```python
from build123d import *

# Parameters (mm, degrees)
SKETCH1_R           = 16
BOSS_EXTRUDE1_DEPTH = 1.6
SKETCH2_W           = 5
SKETCH2_H           = 6.5
BOSS_EXTRUDE2_DEPTH = 1.2
CUT_EXTRUDE1_DEPTH  = 23.683915006
SKETCH4_W           = 11.5
SKETCH4_H           = 5
BOSS_EXTRUDE3_DEPTH = 4.4


with BuildPart() as part:
    # Sketch1 → Boss-Extrude1 (new body)
    with BuildSketch(Plane.XY):
        Circle(SKETCH1_R)
    extrude(amount=BOSS_EXTRUDE1_DEPTH)

    # Sketch2 → Boss-Extrude2 (add)
    with BuildSketch(Plane.XY.offset(1.6)):
        Rectangle(SKETCH2_W, SKETCH2_H)
    extrude(amount=BOSS_EXTRUDE2_DEPTH)

    # Sketch3 → Cut-Extrude1 (cut, through all)
    with BuildSketch(Plane.XY.offset(1.6)):
        with BuildLine():
            Line((-5.656854249, -7.778174593), (-8.838834765, -10.960155108))
            ThreePointArc((-8.838834765, -10.960155108), (-10.960155108, -10.960155108), (-10.960155108, -8.838834765))
            Line((-10.960155108, -8.838834765), (-7.778174593, -5.656854249))
            ThreePointArc((-7.778174593, -5.656854249), (-5.656854249, -5.656854249), (-5.656854249, -7.778174593))
        make_face()
        with BuildLine():
            Line((-9.5, -1.5), (-11.5, -1.5))
            ThreePointArc((-11.5, -1.5), (-13, 0), (-11.5, 1.5))
            Line((-11.5, 1.5), (-9.5, 1.5))
            ThreePointArc((-9.5, 1.5), (-8, 0), (-9.5, -1.5))
        make_face()
        with BuildLine():
            Line((-7.778174593, 5.656854249), (-10.960155108, 8.838834765))
            ThreePointArc((-10.960155108, 8.838834765), (-10.960155108, 10.960155108), (-8.838834765, 10.960155108))
            Line((-8.838834765, 10.960155108), (-5.656854249, 7.778174593))
            ThreePointArc((-5.656854249, 7.778174593), (-5.656854249, 5.656854249), (-7.778174593, 5.656854249))
        make_face()
        with BuildLine():
            Line((5.656854249, 7.778174593), (8.838834765, 10.960155108))
            ThreePointArc((8.838834765, 10.960155108), (10.960155108, 10.960155108), (10.960155108, 8.838834765))
            Line((10.960155108, 8.838834765), (7.778174593, 5.656854249))
            ThreePointArc((7.778174593, 5.656854249), (5.656854249, 5.656854249), (5.656854249, 7.778174593))
        make_face()
        with BuildLine():
            Line((7.778174593, -5.656854249), (10.960155108, -8.838834765))
            ThreePointArc((10.960155108, -8.838834765), (10.960155108, -10.960155108), (8.838834765, -10.960155108))
            Line((8.838834765, -10.960155108), (5.656854249, -7.778174593))
            ThreePointArc((5.656854249, -7.778174593), (5.656854249, -5.656854249), (7.778174593, -5.656854249))
        make_face()
        with BuildLine():
            Line((9.5, 1.5), (11.5, 1.5))
            ThreePointArc((11.5, 1.5), (13, 0), (11.5, -1.5))
            Line((11.5, -1.5), (9.5, -1.5))
            ThreePointArc((9.5, -1.5), (8, 0), (9.5, 1.5))
        make_face()
    extrude(amount=-CUT_EXTRUDE1_DEPTH, mode=Mode.SUBTRACT)

    # Sketch4 → Boss-Extrude3 (add)
    with BuildSketch(Plane(origin=(0, 0, 0), x_dir=(-1, 0, 0), z_dir=(0, 0, -1))):
        with Locations((0, 12)):
            Rectangle(SKETCH4_W, SKETCH4_H)
        with Locations((0, -12)):
            Rectangle(SKETCH4_W, SKETCH4_H)
    extrude(amount=BOSS_EXTRUDE3_DEPTH)


solid = part.part
```
CAD build for the part. Positions are in the model's coordinates, mm. A direction names the side the tool comes from. Round coordinates to 2 decimals unless told otherwise and drop trailing zeros. Order: outer loops, then holes, each group sorted by start corner. A loop starts at its lowest first (then second) coordinate and runs counter-clockwise, first axis right, second up. Notation, with made-up numbers: (-21.75, 76.5) - (11.25, 76.5) arc R28 cw to (11.25, 95.5) - close; hole circle Ø3 at (31.5, 80.25). An arc over 180 degrees is marked (long way). Answer in a Markdown table with one row per item. Add a question column.
(1) Drop flat-ended pins along their axis: pin 1 Ø8 at (x, y) = (1.5, -10.5) entering from +Z; pin 2 Ø1.3 at (x, z) = (-3, -1.5) entering from +Y; pin 3 Ø1 at (y, z) = (-0.5, 2.5) entering from -X; pin 4 Ø3 at (y, z) = (2.5, -2) entering from -X. Give the stop position or say it passes through.
(2) 3-axis set-ups, long thin cutter, end or side, ignore diameter. For faces 1 (the face through (11, -1.5, 1)), 2 (the face through (0, 9.5, -2)), 3 (the face through (5.75, 12, -2)): which of +Z, -Z, +X, -X, +Y, -Y reach the whole face in a straight line?
(3) Band-saw the part on C-C on z = -1. List the corners of the cut face in (x, y).
(4) Band-saw the part on D-D on x = 0. List the corners of the cut face in (y, z), and give its area (3 significant figures).
(5) Band-saw the part on B-B on y = 0. List the corners of the cut face in (x, z), and give its area (3 significant figures).
(6) Band-saw the part on A-A on z = 1. List the corners of the cut face in (x, y).
(7) Mould opens along X. For faces 4 (the face through (0, -9.5, -2)), 5 (the face through (-9.35, 7.23, 0.81)), 6 (the face through (-5.75, -12, -2)) say: +X half, -X half, draft (parallel to the pull), parting line (faces both ways), or undercut.
(8) Probe L1, parallel to Y at x = -2, z = -3.25; L2, parallel to Z at x = 4, y = -5.5; L3, parallel to X at y = 11, z = -0.5. List the from-to ranges inside material, lowest first. Write a range as [from, to].
Data:
| question | item | result |
|---|---|---|
| 1 | pin 1 | stops at z = 1.6 |
| 1 | pin 2 | stops at y = 14.5 |
| 1 | pin 3 | stops at x = -2.5 |
| 1 | pin 4 | passes through |
| 2 | face 1 | +Z, -Z |
| 2 | face 2 | -Z, +X, -X |
| 2 | face 3 | -Z, +X, +Y, -Y |
| 3 | outline | (-5.75, -14.5) - (5.75, -14.5) - (5.75, -9.5) - (-5.75, -9.5) - close; (-5.75, 9.5) - (5.75, 9.5) - (5.75, 14.5) - (-5.75, 14.5) - close |
| 4 | outline | (-16, 0) - (-14.5, 0) - (-14.5, -4.4) - (-9.5, -4.4) - (-9.5, 0) - (9.5, 0) - (9.5, -4.4) - (14.5, -4.4) - (14.5, 0) - (16, 0) - (16, 1.6) - (3.25, 1.6) - (3.25, 2.8) - (-3.25, 2.8) - (-3.25, 1.6) - (-16, 1.6) - close |
| 4 | area | 103 mm^2 |
| 5 | outline | (-16, 0) - (-13, 0) - (-13, 1.6) - (-16, 1.6) - close; (-8, 0) - (8, 0) - (8, 1.6) - (2.5, 1.6) - (2.5, 2.8) - (-2.5, 2.8) - (-2.5, 1.6) - (-8, 1.6) - close; (13, 0) - (16, 0) - (16, 1.6) - (13, 1.6) - close |
| 5 | area | 41.2 mm^2 |
| 6 | outline | circle Ø32 at (0, 0); hole (-11.5, -1.5) - (-9.5, -1.5) arc R1.5 ccw to (-9.5, 1.5) - (-11.5, 1.5) arc R1.5 ccw to start; hole (-10.96, -8.84) arc R1.5 ccw to (-8.84, -10.96) - (-5.66, -7.78) arc R1.5 ccw to (-7.78, -5.66) - close; hole (-10.96, 8.84) - (-7.78, 5.66) arc R1.5 ccw to (-5.66, 7.78) - (-8.84, 10.96) arc R1.5 ccw to start; hole (5.66, -7.78) - (8.84, -10.96) arc R1.5 ccw to (10.96, -8.84) - (7.78, -5.66) arc R1.5 ccw to start; hole (5.66, 7.78) arc R1.5 ccw to (7.78, 5.66) - (10.96, 8.84) arc R1.5 ccw to (8.84, 10.96) - close; hole (9.5, -1.5) - (11.5, -1.5) arc R1.5 ccw to (11.5, 1.5) - (9.5, 1.5) arc R1.5 ccw to start |
| 7 | face 4 | draft |
| 7 | face 5 | undercut |
| 7 | face 6 | -X half |
| 8 | L1 | y = [-14.5, -9.5], [9.5, 14.5] |
| 8 | L2 | z = [0, 1.6] |
| 8 | L3 | x = [-5.75, 5.75] |
